Drawing for the job (mm, zero at the part's lowest x, y, z). A direction names the side the tool comes from. Give positions to 0.01 mm unless a question says otherwise; leave off trailing zeros. Order: outer loops, then holes, each group sorted by start corner. A loop starts at its lowest first (then second) coordinate and runs counter-clockwise, first axis right, second up. Notation, with made-up numbers: (-30.75, 40.5) -> (-0.75, 40.5) arc R22 cw to (-0.75, 64.5) -> close; hole circle Ø2 at (13, 89). An arc over 180 degrees is marked (long way). One line per item, written item: value. Start each with the question number.
(1) Saw through at C-C on x = 3. Give the cut face in (y, z) (1 decimal).
(2) Which spindle directions (+Z, -Z, +X, -X, +Y, -Y) get a long thin tool onto all of the face, cutting with end or side? Do the marked faces 5 and 6. Say none if no direction does.
(3) Pin check, flat tips, straight feed: pin 1 (3 mm diameter, centred on x = 16, z = 75, fed in from -Y); pin 2 (10 mm diameter, centred on x = 23.5, y = 52.5, fed in from -Z) (1 decimal). Stop position of each tip, or through.
(4) Probe line 1 (Z direction, x = 15.5, y = 63.5) (1 decimal). List the from-to ranges inside material, lowest first.
(5) Two-plate mould, pull along X, no slides. Class the marked faces 1, 2, 3 and 4: +X half, -X half, draft (parallel to the pull), parting line (faces both ways), or undercut.
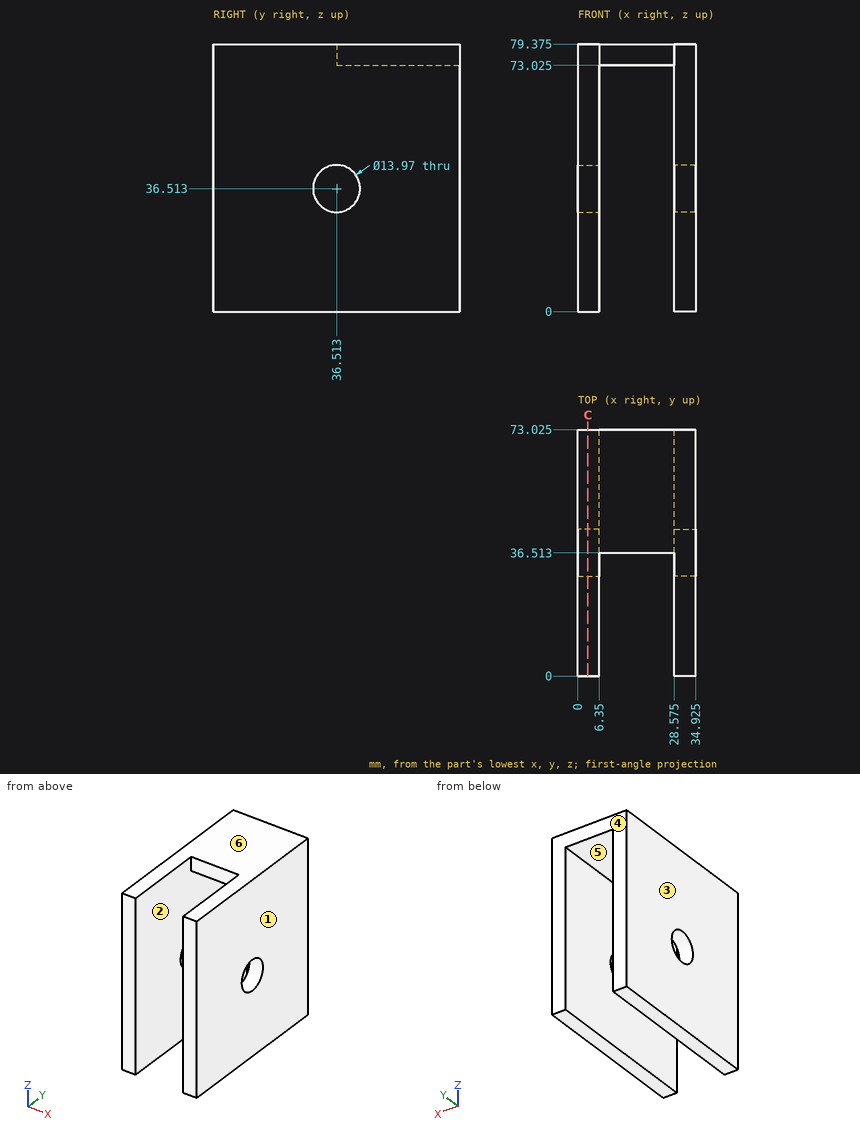
Results below:
1. outline: (0, 0) -> (73, 0) -> (73, 79.4) -> (0, 79.4) -> close; hole circle Ø14 at (36.5, 36.5)
2. face 5: -Z, +Y, -Y
2. face 6: +Z, +X, -X, +Y, -Y
3. pin 1: stops at y = 36.51
3. pin 2: stops at z = 73
4. line 1: z = 73 to 79.4
5. face 1: +X half
5. face 2: undercut
5. face 3: -X half
5. face 4: draft
